Part model, mm, in its own coordinate system. Coordinates: 2 decimals unless noted, no trailing zeros. Order: outer loops, then holes, each group sorted by start corner. A loop starts at its lowest first (then second) coordinate and runs counter-clockwise, first axis right, second up.
1) Pin check, flat tip, straight feed: pin 1 Ø3 at (x, z) = (10.5, -89.5) entering from -Y. Stop position of the tip, or through.
2) Wall check: L1, parallel to X at y = 1.15, z = -89.5; L2, parallel to X at y = 1.6, z = -40; L3, parallel to Z at x = 71.5, y = 2.8. Give the ranges that are in metal, low to high.
3) Mould opens along Z. For faces 1 (the flat face through (59, 1, -100)), 2 (the flat face through (59, 3, -51)), 3 (the cylindrical face through (111.235, 1.521, -10.728)), 4 (the flat face through (59, 1, 0)) say: +Z half, -Z half, draft (parallel to the pull), parting line (faces both ways), or undercut.
4) Cut at A-A (z = -89.5). List the corners of the cut face in (x, y).
```python
from build123d import *

# Parameters (mm, degrees)
SKETCH1_W           = 120
SKETCH1_H           = 100
BOSS_EXTRUDE1_DEPTH = 3
SKETCH2_R           = 1.75
HOLES_SPACERS_DEPTH = 10
HOLES_IMU_REACH     = 158.234
SKETCH3_R           = 1
HOLES_ARDUINO_REACH = 158.234
SKETCH4_R           = 1.8


with BuildPart() as part:
    # Sketch1 → Boss-Extrude1 (new body)
    with BuildSketch(Plane(origin=(0, 0, 0), x_dir=(1, 0, 0), z_dir=(0, 1, 0))):
        with Locations((60, 50)):
            Rectangle(SKETCH1_W, SKETCH1_H)
    extrude(amount=BOSS_EXTRUDE1_DEPTH)

    # Sketch2 → holes_spacers (cut)
    with BuildSketch(Plane(origin=(0, 3, 0), x_dir=(1, 0, 0), z_dir=(0, 1, 0))):
        with Locations(Location((10.5, 89.5, 0), (0, 0, 270))):
            Circle(SKETCH2_R)
        with Locations(Location((109.5, 89.5, 0), (0, 0, 270))):
            Circle(SKETCH2_R)
        with Locations(Location((109.5, 10.5, 0), (0, 0, 270))):
            Circle(SKETCH2_R)
        with Locations(Location((10.5, 10.5, 0), (0, 0, 270))):
            Circle(SKETCH2_R)
    extrude(amount=-HOLES_SPACERS_DEPTH, mode=Mode.SUBTRACT)

    # Sketch3 → holes_IMU (cut, up to next)
    with BuildSketch(Plane(origin=(0, 3, 0), x_dir=(1, 0, 0), z_dir=(0, 1, 0)), mode=Mode.PRIVATE) as holes_imu_sk1:
        with Locations(Location((35, 60, 0), (0, 0, 270))):
            Circle(SKETCH3_R)
    holes_imu_tool1 = extrude(holes_imu_sk1.sketch, amount=-HOLES_IMU_REACH, mode=Mode.PRIVATE) & part.part
    # Sketch3 → holes_IMU (cut, up to next)
    with BuildSketch(Plane(origin=(0, 3, 0), x_dir=(1, 0, 0), z_dir=(0, 1, 0)), mode=Mode.PRIVATE) as holes_imu_sk2:
        with Locations(Location((55, 60, 0), (0, 0, 270))):
            Circle(SKETCH3_R)
    holes_imu_tool2 = extrude(holes_imu_sk2.sketch, amount=-HOLES_IMU_REACH, mode=Mode.PRIVATE) & part.part
    # Sketch3 → holes_IMU (cut, up to next)
    with BuildSketch(Plane(origin=(0, 3, 0), x_dir=(1, 0, 0), z_dir=(0, 1, 0)), mode=Mode.PRIVATE) as holes_imu_sk3:
        with Locations(Location((55, 40, 0), (0, 0, 270))):
            Circle(SKETCH3_R)
    holes_imu_tool3 = extrude(holes_imu_sk3.sketch, amount=-HOLES_IMU_REACH, mode=Mode.PRIVATE) & part.part
    # Sketch3 → holes_IMU (cut, up to next)
    with BuildSketch(Plane(origin=(0, 3, 0), x_dir=(1, 0, 0), z_dir=(0, 1, 0)), mode=Mode.PRIVATE) as holes_imu_sk4:
        with Locations(Location((35, 40, 0), (0, 0, 270))):
            Circle(SKETCH3_R)
    holes_imu_tool4 = extrude(holes_imu_sk4.sketch, amount=-HOLES_IMU_REACH, mode=Mode.PRIVATE) & part.part
    add(holes_imu_tool1.solids().sort_by_distance((35, 3, -60))[0], mode=Mode.SUBTRACT)
    add(holes_imu_tool2.solids().sort_by_distance((55, 3, -60))[0], mode=Mode.SUBTRACT)
    add(holes_imu_tool3.solids().sort_by_distance((55, 3, -40))[0], mode=Mode.SUBTRACT)
    add(holes_imu_tool4.solids().sort_by_distance((35, 3, -40))[0], mode=Mode.SUBTRACT)

    # Sketch4 → holes_arduino (cut, up to next)
    with BuildSketch(Plane(origin=(0, 3, 0), x_dir=(1, 0, 0), z_dir=(0, 1, 0)), mode=Mode.PRIVATE) as holes_arduino_sk1:
        with Locations(Location((66.389668811, 76.207441627, 0), (0, 0, 270))):
            Circle(SKETCH4_R)
    holes_arduino_tool1 = extrude(holes_arduino_sk1.sketch, amount=-HOLES_ARDUINO_REACH, mode=Mode.PRIVATE) & part.part
    # Sketch4 → holes_arduino (cut, up to next)
    with BuildSketch(Plane(origin=(0, 3, 0), x_dir=(1, 0, 0), z_dir=(0, 1, 0)), mode=Mode.PRIVATE) as holes_arduino_sk2:
        with Locations(Location((112.329668811, 75.287441627, 0), (0, 0, 270))):
            Circle(SKETCH4_R)
    holes_arduino_tool2 = extrude(holes_arduino_sk2.sketch, amount=-HOLES_ARDUINO_REACH, mode=Mode.PRIVATE) & part.part
    # Sketch4 → holes_arduino (cut, up to next)
    with BuildSketch(Plane(origin=(0, 3, 0), x_dir=(1, 0, 0), z_dir=(0, 1, 0)), mode=Mode.PRIVATE) as holes_arduino_sk3:
        with Locations(Location((97.519668811, 24.837441627, 0), (0, 0, 270))):
            Circle(SKETCH4_R)
    holes_arduino_tool3 = extrude(holes_arduino_sk3.sketch, amount=-HOLES_ARDUINO_REACH, mode=Mode.PRIVATE) & part.part
    # Sketch4 → holes_arduino (cut, up to next)
    with BuildSketch(Plane(origin=(0, 3, 0), x_dir=(1, 0, 0), z_dir=(0, 1, 0)), mode=Mode.PRIVATE) as holes_arduino_sk4:
        with Locations(Location((70.779668811, 24.837441627, 0), (0, 0, 270))):
            Circle(SKETCH4_R)
    holes_arduino_tool4 = extrude(holes_arduino_sk4.sketch, amount=-HOLES_ARDUINO_REACH, mode=Mode.PRIVATE) & part.part
    add(holes_arduino_tool1.solids().sort_by_distance((66.389669, 3, -76.207442))[0], mode=Mode.SUBTRACT)
    add(holes_arduino_tool2.solids().sort_by_distance((112.329669, 3, -75.287442))[0], mode=Mode.SUBTRACT)
    add(holes_arduino_tool3.solids().sort_by_distance((97.519669, 3, -24.837442))[0], mode=Mode.SUBTRACT)
    add(holes_arduino_tool4.solids().sort_by_distance((70.779669, 3, -24.837442))[0], mode=Mode.SUBTRACT)


solid = part.part
```
Geometry check:
1. pin 1: passes through
2. L1: x = 0 to 8.75, 12.25 to 107.75, 111.25 to 120
2. L2: x = 0 to 34, 36 to 54, 56 to 120
2. L3: z = -100 to -26.49, -23.19 to 0
3. face 1: -Z half
3. face 2: draft
3. face 3: undercut
3. face 4: +Z half
4. outline: (0, 0) - (8.75, 0) - (8.75, 3) - (0, 3) - close; (12.25, 0) - (107.75, 0) - (107.75, 3) - (12.25, 3) - close; (111.25, 0) - (120, 0) - (120, 3) - (111.25, 3) - close
